from build123d import *

# Parameters (mm, degrees)
SKETCH_1_W             = 4.9
SKETCH_1_H             = 12
EXTRUDE_1_DEPTH        = 17
SKETCH_2_W             = 1.2
SKETCH_2_H             = 5
CUT_EXTRUDE_1_DEPTH    = 18
FILLET_1_R             = 0.5
HOLE_WIZARD_M2_1_D     = 1.6
HOLE_WIZARD_M2_1_DEPTH = 2.2
HOLE_WIZARD_M2_1_TIP   = 0.480688495


with BuildPart() as part:
    # 草图1 → 凸台-拉伸1 (new body)
    with BuildSketch(Plane.XY):
        Rectangle(SKETCH_1_W, SKETCH_1_H)
    extrude(amount=EXTRUDE_1_DEPTH)

    # 草图2 → 切除-拉伸1 (cut, through all)
    with BuildSketch(Plane.XY.offset(17)):
        with Locations((-1.85, 0)):
            Rectangle(SKETCH_2_W, SKETCH_2_H)
    extrude(amount=-CUT_EXTRUDE_1_DEPTH, mode=Mode.SUBTRACT)

    # 圆角1
    fillet_1_edges = [part.edges().sort_by_distance(p)[0] for p in [
        (2.45, 6, 8.5),
        (2.45, -6, 8.5),
    ]]
    fillet(fillet_1_edges, radius=FILLET_1_R)

    # M2 螺纹孔1
    with Locations(Plane(origin=(2.45, 0, 0), x_dir=(0, 0, -1), z_dir=(1, 0, 0))):
        with Locations((-8.5, 4), (-8.5, -4)):
            Hole(HOLE_WIZARD_M2_1_D / 2, depth=HOLE_WIZARD_M2_1_DEPTH)
            with Locations((0, 0, -(HOLE_WIZARD_M2_1_DEPTH + HOLE_WIZARD_M2_1_TIP / 2))):  # 118° drill point
                Cone(0, HOLE_WIZARD_M2_1_D / 2, HOLE_WIZARD_M2_1_TIP, mode=Mode.SUBTRACT)


solid = part.part
Geometry: final body of the model. Coordinates: model frame, mm. A direction names the side the tool comes from. Give positions to 0.01 mm unless a question says otherwise; leave off trailing zeros. Order: outer loops, then holes, each group sorted by start corner. A loop starts at its lowest first (then second) coordinate and runs counter-clockwise, first axis right, second up. Notation, with made-up numbers: (-12.5, 34.5) -> (6.5, 34.5) arc R18 cw to (6.5, 48.5) -> close; hole circle Ø10 at (27, 61). An arc over 180 degrees is marked (long way). Answer as a JSON object with one key per item and string values.
Q1. Section C-C (y = 0.25). Output: boundary loops of the cut face in (x, z), plus the area to 3 significant figures.
Entries:
{"outline": "(-1.25, 0) -> (2.45, 0) -> (2.45, 17) -> (-1.25, 17) -> close", "area": "62.9 mm^2"}
Q2. Material intervals for probe 1 along Y at (x, z) = (1.7, 8.5); probe 2 along Y at (x, z) = (1.15, 8); probe 3 along Y at (x, z) = (-1.4, 4), sorted ascending.
Entries:
{"probe 1": "y = -6 to -4.8, -3.2 to 3.2, 4.8 to 6", "probe 2": "y = -6 to -4.62, -3.38 to 3.38, 4.62 to 6", "probe 3": "y = -6 to -2.5, 2.5 to 6"}
Q3. First-contact query: pin 1 (2.5 mm diameter, centred on y = 0, z = 12.5, fed in from -X); pin 2 (1.4 mm diameter, centred on y = -4, z = 8.5, fed in from +X). Flat tips, straight axial feed; report the tip coordinate or a pass-through.
Entries:
{"pin 1": "stops at x = -1.25", "pin 2": "stops at x = 0.19"}
Q4. Section B-B (x = 0.95). Output: boundary loops of the cut face in (y, z), plus the area to 3 significant figures.
Entries:
{"outline": "(-6, 0) -> (6, 0) -> (6, 17) -> (-6, 17) -> close; hole circle Ø1.6 at (-4, 8.5); hole circle Ø1.6 at (4, 8.5)", "area": "200 mm^2"}
Q5. Draft query along Z for faces 4 (the conical face through (-0.15, -4.08, 8.61)), 5 (the conical face through (-0.15, 3.88, 8.44)), 6 (the flat face through (-2, -2.5, 9)), 7 (the flat face through (0, 0, 0)). Return one class per face: released by +Z, released by -Z, zero draft, split by the parting line, or undercut.
Entries:
{"face 4": "undercut", "face 5": "undercut", "face 6": "zero draft", "face 7": "released by -Z"}
Q6. Section A-A (z = 14.25). Output: boundary loops of the cut face in (x, y).
Entries:
{"outline": "(-2.45, -6) -> (1.95, -6) arc R0.5 ccw to (2.45, -5.5) -> (2.45, 5.5) arc R0.5 ccw to (1.95, 6) -> (-2.45, 6) -> (-2.45, 2.5) -> (-1.25, 2.5) -> (-1.25, -2.5) -> (-2.45, -2.5) -> close"}
Q7. Access query for faces 1 (the cylindrical face through (1.3, -4, 7.7)), 2 (the flat face through (-1.25, 0, 9)), 3 (the flat face through (0, 6, 8)). Directions: +Z, -Z, +X, -X, +Y, -Y. A direction counts if a zero-diameter tool reaches every point of the face in a straight line with its end or side. Return the directions, or none.
Entries:
{"face 1": "+X", "face 2": "+Z, -Z, -X", "face 3": "+Z, -Z, +X, -X, +Y"}
